Verification items for the finished model (mm, model axes). Round coordinates to 2 decimals unless told otherwise and drop trailing zeros. Order: outer loops, then holes, each group sorted by start corner. A loop starts at its lowest first (then second) coordinate and runs counter-clockwise, first axis right, second up. Notation, with made-up numbers: (-4, 73) -> (42, 73) arc R23 cw to (42, 101) -> close; hole circle Ø5 at (11, 87.5). An arc over 180 degrees is marked (long way). Put each result on its own line as item: value.
from build123d import *

# Parameters (mm, degrees)
F2_R = 2.54
F3_R = 5.08


with BuildPart() as f1:
    # F0 (on Front) → F1 (revolve)
    with BuildSketch(Plane.XZ):
        Polygon((0, 247.65), (0, 0), (23.495, 0), (23.495, 209.55), (14.2875, 247.65), align=None)
    revolve(axis=Axis((0, 0, 5.152837), (0, 0, 1)))

    # F2
    f2_edges = [f1.edges().sort_by_distance(p)[0] for p in [
        (-14.2875, 0, 247.65),
    ]]
    fillet(f2_edges, radius=F2_R)

    # F3
    f3_edges = [f1.edges().sort_by_distance(p)[0] for p in [
        (-23.495, 0, 209.55),
    ]]
    fillet(f3_edges, radius=F3_R)


solid = f1.part
Item 1: Material ranges on L1, parallel to X at y = -1, z = 68; L2, parallel to X at y = 1.5, z = 165; L3, parallel to Y at x = -10, z = 68, recorded low to high. Write a range as [from, to].
Check sheet entries:
L1: x = [-23.47, 23.47]
L2: x = [-23.45, 23.45]
L3: y = [-21.26, 21.26]
Item 2: Section check A-A on z = 138.5. Record the boundary of the cut face in (x, y) (3 decimals).
Check sheet entries:
outline: circle Ø46.99 at (0, 0)
Item 3: Gauge pin test, flat ends, axial feed: pin 1 Ø5 at (x, z) = (7, 155) entering from -Y; pin 2 Ø10 at (y, z) = (15.5, 127) entering from -X; pin 3 Ø5 at (x, z) = (-13.5, 55.5) entering from +Y. Record the tip position at first contact, or that the pin passes through.
Check sheet entries:
pin 1: stops at y = -23.06
pin 2: stops at x = -21.02
pin 3: stops at y = 20.76
